Check sheet for the drawn part. Datum: minimum x, y, z corner. Units: mm. Coordinates: 2 decimals unless noted, no trailing zeros. Write each loop counter-clockwise with the first axis right and the second up, starting at its lowest first coordinate (ties: lowest second). Pieces come first, ordered by that corner, then holes. Notation, with made-up numbers: (-27.75, -10) -> (3.25, -10) arc R12 ccw to (3.25, -5) -> close; hole circle Ø11 at (45, 87). An arc over 180 degrees is marked (long way). Answer in a Markdown table with one row per item.
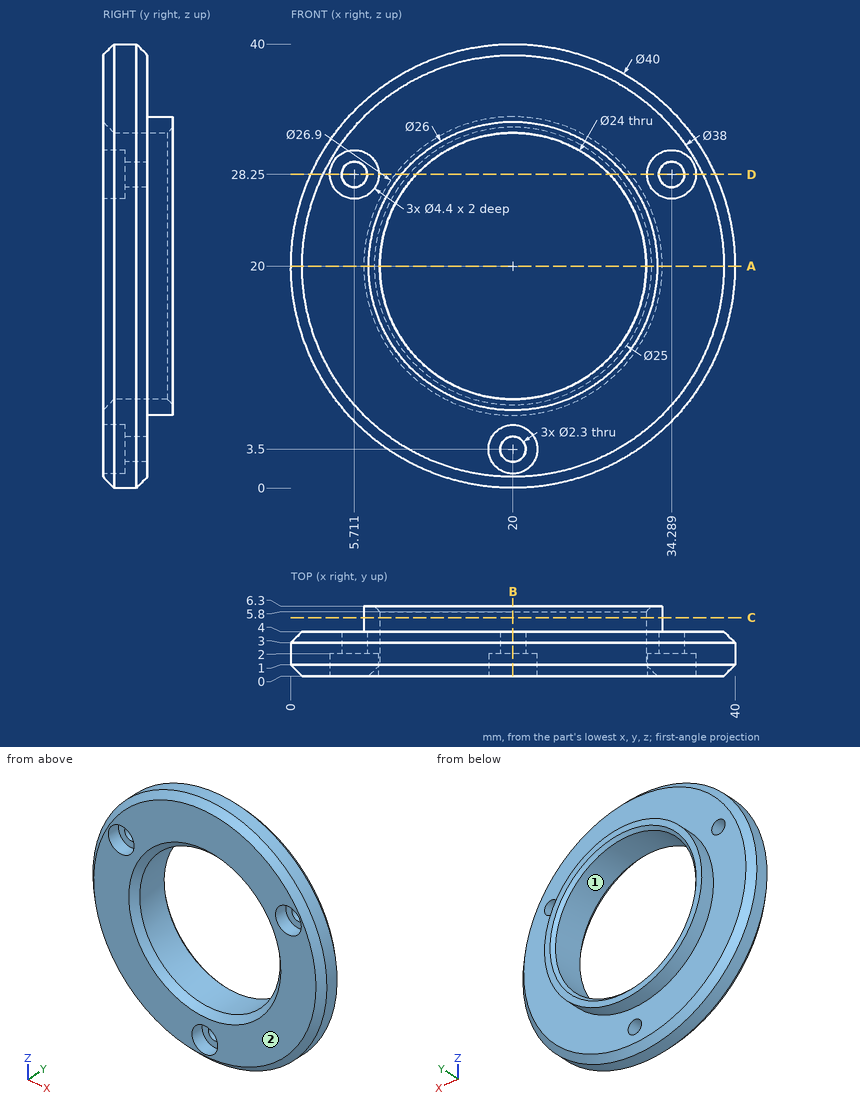
1. Go/stop test with flat-tipped pins: pin 1 (2 mm diameter, centred on x = 34.5, y = 3.5, fed in from +Z); pin 2 (3 mm diameter, centred on y = 5, z = 23, fed in from +X) (1 decimal); pin 3 (3.5 mm diameter, centred on x = 5.71, z = 28.25, fed in from +Y); pin 4 (19 mm diameter, centred on x = 20, z = 20, fed in from -Y). Record where each tip stops, or that it passes through.
Findings below:
| item | result |
|---|---|
| pin 1 | stops at z = 34.63 |
| pin 2 | stops at x = 39.3 |
| pin 3 | stops at y = 4 |
| pin 4 | passes through |
2. Sectioned sample at D-D, the plane z = 28.25. Count the separate pieces of the cut face and the enclosed holes in it.
Findings below:
| item | result |
|---|---|
| separate pieces | 4 |
| enclosed holes | 0 |
3. Sectioned sample at A-A, the plane z = 20. Record the cut outline in (x, y).
Findings below:
| item | result |
|---|---|
| outline | (0, 1) -> (1, 0) -> (7, 0) -> (8, 1) -> (8, 5.8) -> (7.5, 6.3) -> (6.55, 6.3) -> (6.55, 4) -> (1, 4) -> (0, 3) -> close; (32, 1) -> (33, 0) -> (39, 0) -> (40, 1) -> (40, 3) -> (39, 4) -> (33.45, 4) -> (33.45, 6.3) -> (32.5, 6.3) -> (32, 5.8) -> close |
4. Sectioned sample at B-B, the plane x = 20. Record the cut outline in (y, z).
Findings below:
| item | result |
|---|---|
| outline | (0, 1) -> (1, 0) -> (3, 0) -> (4, 1) -> (4, 2.35) -> (2, 2.35) -> (2, 1.3) -> (0, 1.3) -> close; (0, 5.7) -> (2, 5.7) -> (2, 4.65) -> (4, 4.65) -> (4, 6.55) -> (6.3, 6.55) -> (6.3, 7.5) -> (5.8, 8) -> (1, 8) -> (0, 7) -> close; (0, 33) -> (1, 32) -> (5.8, 32) -> (6.3, 32.5) -> (6.3, 33.45) -> (4, 33.45) -> (4, 39) -> (3, 40) -> (1, 40) -> (0, 39) -> close |
5. Sectioned sample at C-C, the plane y = 5.25. Record the cut outline in (x, z), and give its area (3 significant figures).
Findings below:
| item | result |
|---|---|
| outline | circle Ø26.9 at (20, 20); hole circle Ø24 at (20, 20) |
| area | 116 mm² |
6. Release check for a two-part mould opening along X. For the marked faces 1 and 2 record: released by +X, released by -X, zero draft, split by the parting line, or undercut.
Findings below:
| item | result |
|---|---|
| face 1 | undercut |
| face 2 | zero draft |
7. Material ranges on probe 1 along X at (y, z) = (3.05, 28.25) (1 decimal); probe 2 along X at (y, z) = (0.5, 28.25); probe 3 along Y at (x, z) = (5, 23), recorded low to high. Write a range as from..to.
Findings below:
| item | result |
|---|---|
| probe 1 | x = 1.8..4.6, 6.9..11.3, 28.7..33.1, 35.4..38.2 |
| probe 2 | x = 2.33..3.51, 7.91..10.61, 29.39..32.09, 36.49..37.67 |
| probe 3 | y = 0..4 |
